Could you check a few things on this model? Use its own coordinates, in mm. A direction names the side the tool comes from. Give positions to 0.01 mm unless a question says otherwise; leave off trailing zeros. Loops run counter-clockwise (first coordinate to the right, second up) from the corner with the lowest first, then second, coordinate; pieces in that order, holes last. Notation, with made-up numbers: (-9, 45) - (21, 45) arc R10 ccw to (21, 53) - close; hole circle Ø4 at (68.25, 88.25). An arc over 180 degrees is marked (long way). One line per item, written item: value. Start each with the question number.
Q1. I want a section at D-D (y = 11.5). Please give me the cut outline in (x, z).
Q2. For faces 4 (the face through (0, 0, 95)), 5 (the face through (0, 0, 100)), which set-ups out of +Z, -Z, +X, -X, +Y, -Y let a thin tool reach every point of the face, with its end or its side?
Q3. I'm going to push flat-ended pins straight in: P1, Ø1, axis at x = 0, y = -11.5, coming from the -Z side; P2, Ø6, axis at x = 0, y = -3.5, coming from the -Z side; P3, Ø4, axis at x = 3.5, z = 79.5, coming from the +Y side. Where does each tip first touch, or does it pass through?
Q4. I want a section at A-A (x = 0). Please give me the cut outline in (y, z).
Q5. If we mould it in two halves opening along X, with no side actions, what happens to faces 1 (the face through (-10.316, -7.91, 49.3)), 2 (the face through (12, 0, 5)), 3 (the face through (-10, 3, 0))? For each: released by +X, released by -X, zero draft, split by the parting line, or undercut.
Q6. If I drill on line 1 (Y direction, x = 0, z = 66.5); line 2 (Y direction, x = 0, z = 3.9), over which ranges is the centre line in solid material (lowest first)? Write a range as from..to.
Q7. I want a section at C-C (z = 21.5). Please give me the cut outline in (x, y), then the cut area to 3 significant figures.
```python
from build123d import *

# Parameters (mm, degrees)
SKETCH_1_R          = 13
SKETCH_1_R_2        = 10
EXTRUDE_1_DEPTH     = 100
EXTRUDE_START       = -5
SKETCH_2_R          = 13
EXTRUDE_2_DEPTH     = 5
SKETCH_3_R          = 1
CUT_EXTRUDE_1_DEPTH = 5


with BuildPart() as part:
    # 草图1 → 凸台-拉伸1 (new body)
    with BuildSketch(Plane.XY):
        Circle(SKETCH_1_R)
        Circle(SKETCH_1_R_2, mode=Mode.SUBTRACT)
    extrude(amount=EXTRUDE_1_DEPTH)

    # 草图2 → 凸台-拉伸2 (add)
    with BuildSketch(Plane.XY.offset(100).offset(EXTRUDE_START)):
        Circle(SKETCH_2_R)
    extrude(amount=EXTRUDE_2_DEPTH)

    # 草图3 → 切除-拉伸1 (cut)
    with BuildSketch(Plane(origin=(0, 0, 0), x_dir=(-1, 0, 0), z_dir=(0, 0, -1))):
        with Locations((0, 11.5)):
            Circle(SKETCH_3_R)
        with Locations((11.5, 0)):
            Circle(SKETCH_3_R)
        with Locations((0, -11.5)):
            Circle(SKETCH_3_R)
        with Locations((-11.5, 0)):
            Circle(SKETCH_3_R)
    extrude(amount=-CUT_EXTRUDE_1_DEPTH, mode=Mode.SUBTRACT)


solid = part.part
```
Worked answers:
1. outline: (-6.06, 0) - (-1, 0) - (-1, 5) - (1, 5) - (1, 0) - (6.06, 0) - (6.06, 100) - (-6.06, 100) - close
2. face 4: -Z
2. face 5: +Z, +X, -X, +Y, -Y
3. P1: stops at z = 5
3. P2: stops at z = 95
3. P3: stops at y = 12.91
4. outline: (-13, 0) - (-12.5, 0) - (-12.5, 5) - (-10.5, 5) - (-10.5, 0) - (-10, 0) - (-10, 95) - (10, 95) - (10, 0) - (10.5, 0) - (10.5, 5) - (12.5, 5) - (12.5, 0) - (13, 0) - (13, 100) - (-13, 100) - close
5. face 1: split by the parting line
5. face 2: undercut
5. face 3: zero draft
6. line 1: y = -13..-10, 10..13
6. line 2: y = -13..-12.5, -10.5..-10, 10..10.5, 12.5..13
7. outline: circle Ø26 at (0, 0); hole circle Ø20 at (0, 0)
7. area: 217 mm²
